```python
from build123d import *

# Parameters (mm, degrees)
ESQUISSE1_W             = 60
ESQUISSE1_H             = 30
BOSS_EXTRU_1_DEPTH      = 5
ESQUISSE2_R             = 8
ENL_V_MAT_EXTRU_1_DEPTH = 5
ESQUISSE4_W             = 10
ESQUISSE4_H             = 5
BOSS_EXTRU_2_DEPTH      = 10
ESQUISSE6_R             = 2
ENL_V_MAT_EXTRU_2_DEPTH = 10
BOSS_EXTRU_3_DEPTH      = 2
SYM_TRIE4_COPY_1_DEPTH  = 2
ENL_V_MAT_EXTRU_3_DEPTH = 68.823299831


with BuildPart() as part:
    # Esquisse1 → Boss.-Extru.1 (new body)
    with BuildSketch(Plane.XY):
        with Locations((30, 15)):
            Rectangle(ESQUISSE1_W, ESQUISSE1_H)
    extrude(amount=BOSS_EXTRU_1_DEPTH)

    # Esquisse2 → Enlèv. mat.-Extru.1 (cut)
    with BuildSketch(Plane.XY.offset(5)):
        with Locations((30, 15)):
            Circle(ESQUISSE2_R)
    extrude(amount=-ENL_V_MAT_EXTRU_1_DEPTH, mode=Mode.SUBTRACT)

    # Esquisse4 → Boss.-Extru.2 (add)
    with BuildSketch(Plane.XY.offset(5)):
        with Locations((55, 2.5)):
            Rectangle(ESQUISSE4_W, ESQUISSE4_H)
    boss_extru_2 = extrude(amount=BOSS_EXTRU_2_DEPTH)

    # Symétrie1: Boss.-Extru.2 across plane
    add(boss_extru_2.mirror(Plane(origin=(30, 0, 0), x_dir=(0, 0, 1), z_dir=(1, 0, 0))))

    # Esquisse6 → Enlèv. mat.-Extru.2 (cut)
    with BuildSketch(Plane(origin=(0, 5, 0), x_dir=(1, 0, 0), z_dir=(0, 1, 0))):
        with Locations(Location((5, -10, 0), (0, 0, 180))):
            Circle(ESQUISSE6_R)
    enl_v_mat_extru_2 = extrude(amount=-ENL_V_MAT_EXTRU_2_DEPTH, mode=Mode.SUBTRACT)

    # Symétrie2: Enlèv. mat.-Extru.2 across plane
    add(enl_v_mat_extru_2.mirror(Plane(origin=(30, 0, 0), x_dir=(0, 0, 1), z_dir=(1, 0, 0))), mode=Mode.SUBTRACT)

    # Esquisse13 → Boss.-Extru.3 (add)
    with BuildSketch(Plane.ZY):
        Polygon((15, 5), (5, 11.605187872), (5, 5), align=None)
    boss_extru_3 = extrude(amount=-BOSS_EXTRU_3_DEPTH)

    # Symétrie3: Boss.-Extru.3 across plane
    add(boss_extru_3.mirror(Plane.ZY.offset(-5)))

    # Symétrie4: Boss.-Extru.3 across plane
    add(boss_extru_3.mirror(Plane(origin=(30, 0, 0), x_dir=(0, 0, 1), z_dir=(1, 0, 0))))

    # Symétrie4 copy 1 sketch → Symétrie4 copy 1 (add)
    with BuildSketch(Plane.ZY.offset(-50)):
        Polygon((15, 5), (5, 11.605187872), (5, 5), align=None)
    extrude(amount=-SYM_TRIE4_COPY_1_DEPTH)

    # Esquisse14 → Enlèv. mat.-Extru.3 (cut, through all)
    with BuildSketch(Plane.XY.offset(5)):
        Polygon((20, 30), (0, 20), (0, 30), align=None)
    enl_v_mat_extru_3 = extrude(amount=-ENL_V_MAT_EXTRU_3_DEPTH, mode=Mode.SUBTRACT)

    # Symétrie5: Enlèv. mat.-Extru.3 across plane
    add(enl_v_mat_extru_3.mirror(Plane(origin=(30, 0, 0), x_dir=(0, 0, 1), z_dir=(1, 0, 0))), mode=Mode.SUBTRACT)


solid = part.part
```
The listing builds one solid part. Answer for the finished solid, in the listing's coordinates (mm). A direction names the side the tool comes from. Coordinates: 2 decimals unless noted, no trailing zeros. Write each loop counter-clockwise with the first axis right and the second up, starting at its lowest first coordinate (ties: lowest second). Pieces come first, ordered by that corner, then holes. Notation, with made-up numbers: M -22.5,47.5 L -11.5,47.5 A15 ccw -11.5,67.5 Z; hole C 65,29 d9. An arc over 180 degrees is marked long. Use a Markdown table: item, result. Add a question column.
1. Section B-B (y = 15) is taken. Give the vertices of the cut face in (x, z), plus the area to 3 significant figures.
2. Section A-A (x = 30) is taken. Give the vertices of the cut face in (y, z), plus the area to 3 significant figures.
3. Which of the six approach directions +Z, -Z, +X, -X, +Y, -Y give full straight-line access (tool end or side, diameter ignored) to faces 1 (the flat face through (5, 5, 12.2)), 2 (the flat face through (50, 5, 9)), 3 (the flat face through (0.986, 8.256, 10.07))?
4. Given P1, Ø5, axis at x = 41.5, z = 9, coming from the -Y side; P2, Ø4, axis at x = 15.5, y = 10.5, coming from the -Z side; P3, Ø15, axis at x = 19.5, y = 11, coming from the +Z side; P4, Ø1, axis at y = 22.5, z = 1.5, coming from the -X side, each flat-ended and moving along its own axis, determine where each tip first touches the part or whether it passes through.
5. Section C-C (z = 6.75) is taken. Give the vertices of the cut face in (x, y), plus the area to 3 significant figures.
6. For a pull along Z with two mould halves and no side action, classify faces 4 (the cylindrical face through (5, 3, 12)), 5 (the flat face through (50.986, 8.256, 10.07)), 6 (the flat face through (30, 5, 0)), 7 (the flat face through (60, 8, 6)) as +Z half, -Z half, draft (parallel to the pull), parting line (faces both ways), or undercut.
7. Section D-D (z = 10) is taken. Give the vertices of the cut face in (x, y), plus the area to 3 significant figures.
8. Straight lines are drawn through the part: line 1 along X through (y, z) = (7, 6.5); line 2 along Z through (x, y) = (55, 1.15); line 3 along X through (y, z) = (16.75, 3.75). For each, find the intervals that lie inside material, in ascending order. Write a range as [from, to].
Data:
| question | item | result |
|---|---|---|
| 1 | outline | M 0,0 L 22,0 L 22,5 L 0,5 Z; M 38,0 L 60,0 L 60,5 L 38,5 Z |
| 1 | area | 220 mm2 |
| 2 | outline | M 0,0 L 7,0 L 7,5 L 0,5 Z; M 23,0 L 30,0 L 30,5 L 23,5 Z |
| 2 | area | 70.0 mm2 |
| 3 | face 1 | +Z, +Y |
| 3 | face 2 | +Z, +Y, -Y |
| 3 | face 3 | +Z, +X, -X, +Y |
| 4 | P1 | passes through |
| 4 | P2 | stops at z = 0 |
| 4 | P3 | stops at z = 5 |
| 4 | P4 | stops at x = 4 |
| 5 | outline | M 0,0 L 10,0 L 10,10.45 L 8,10.45 L 8,5 L 2,5 L 2,10.45 L 0,10.45 Z; M 50,0 L 60,0 L 60,10.45 L 58,10.45 L 58,5 L 52,5 L 52,10.45 L 50,10.45 Z |
| 5 | area | 144 mm2 |
| 6 | face 4 | undercut |
| 6 | face 5 | +Z half |
| 6 | face 6 | -Z half |
| 6 | face 7 | draft |
| 7 | outline | M 0,0 L 3,0 L 3,5 L 2,5 L 2,8.3 L 0,8.3 Z; M 7,0 L 10,0 L 10,8.3 L 8,8.3 L 8,5 L 7,5 Z; M 50,0 L 53,0 L 53,5 L 52,5 L 52,8.3 L 50,8.3 Z; M 57,0 L 60,0 L 60,8.3 L 58,8.3 L 58,5 L 57,5 Z |
| 7 | area | 86.4 mm2 |
| 8 | line 1 | x = [0, 2], [8, 10], [50, 52], [58, 60] |
| 8 | line 2 | z = [0, 8], [12, 15] |
| 8 | line 3 | x = [0, 22.19], [37.81, 60] |
